from build123d import *

# Parameters (mm, degrees)
MODEL_R                 = 1.5
SALIENTE_EXTRUIR1_DEPTH = 3


with BuildPart() as part:
    # Model → Saliente-Extruir1 (new body)
    with BuildSketch(Plane.XY):
        Polygon((-105.943383637, 105.556539338), (-105.943383637, 51.556539338), (-51.943383637, 51.556539338), align=None)
        with Locations((-101.443383637, 92.056539338)):
            Circle(MODEL_R, mode=Mode.SUBTRACT)
        with Locations((-101.443383637, 83.056539338)):
            Circle(MODEL_R, mode=Mode.SUBTRACT)
        with Locations((-92.443383637, 83.056539338)):
            Circle(MODEL_R, mode=Mode.SUBTRACT)
        with Locations((-101.443383637, 74.056539338)):
            Circle(MODEL_R, mode=Mode.SUBTRACT)
        with Locations((-92.443383637, 74.056539338)):
            Circle(MODEL_R, mode=Mode.SUBTRACT)
        with Locations((-83.443383637, 74.056539338)):
            Circle(MODEL_R, mode=Mode.SUBTRACT)
        with Locations((-101.443383637, 65.056539338)):
            Circle(MODEL_R, mode=Mode.SUBTRACT)
        with Locations((-92.443383637, 65.056539338)):
            Circle(MODEL_R, mode=Mode.SUBTRACT)
        with Locations((-83.443383637, 65.056539338)):
            Circle(MODEL_R, mode=Mode.SUBTRACT)
        with Locations((-74.443383637, 65.056539338)):
            Circle(MODEL_R, mode=Mode.SUBTRACT)
        with Locations((-101.443383637, 56.056539338)):
            Circle(MODEL_R, mode=Mode.SUBTRACT)
        with Locations((-92.443383637, 56.056539338)):
            Circle(MODEL_R, mode=Mode.SUBTRACT)
        with Locations((-83.443383637, 56.056539338)):
            Circle(MODEL_R, mode=Mode.SUBTRACT)
        with Locations((-74.443383637, 56.056539338)):
            Circle(MODEL_R, mode=Mode.SUBTRACT)
        with Locations((-65.443383637, 56.056539338)):
            Circle(MODEL_R, mode=Mode.SUBTRACT)
    extrude(amount=SALIENTE_EXTRUIR1_DEPTH)


solid = part.part
Can you work these out from the model? Positions are in its coordinate system, mm. Round coordinates to 2 decimals unless told otherwise and drop trailing zeros. Order: outer loops, then holes, each group sorted by start corner. A loop starts at its lowest first (then second) coordinate and runs counter-clockwise, first axis right, second up. Notation, with made-up numbers: (82, -1.5) -> (93, -1.5) arc R14 ccw to (93, 20.5) -> close; hole circle Ø10 at (8.5, -36.5). An arc over 180 degrees is marked (long way). Write each question's results on one line, items separated by ' | '. Start each with the question number.
Item 1: If we section it at C-C, the plane z = 1.65: State how many separate pieces and enclosed holes the cut face has, then the cut area to 3 significant figures.
Item 2: Thinking about a two-plate mould opening in X: for faces 1 (the flat face through (-91, 67, 0)), 2 (the flat face through (-78.565, 78.179, 1.479)), 3 (the cylindrical face through (-100.8, 90.7, 1.5)), which applies, +X half, -X half, draft (parallel to the pull), parting line (faces both ways), or undercut?
Item 3: If we section it at A-A, the plane x = -65.5: Write out the boundary of the cut face in (y, z), then the cut area to 3 significant figures.
Item 4: If we section it at D-D, the plane x = -102: Write out the boundary of the cut face in (y, z).
Item 5: If we section it at B-B, the plane x = -74.5: Write out the boundary of the cut face in (y, z).
Item 6: Please list where these lines run through material, in increasing order: L1, parallel to X at y = 82, z = 0.3; L2, parallel to Y at x = -73.5, z = 1.4; L3, parallel to X at y = 74, z = 1.7.
Results:
1) separate pieces: 1 | enclosed holes: 15 | area: 1,350 mm2
2) face 1: draft | face 2: +X half | face 3: undercut
3) outline: (51.56, 0) -> (54.56, 0) -> (54.56, 3) -> (51.56, 3) -> close; (57.56, 0) -> (65.11, 0) -> (65.11, 3) -> (57.56, 3) -> close | area: 31.7 mm2
4) outline: (51.56, 0) -> (54.66, 0) -> (54.66, 3) -> (51.56, 3) -> close; (57.45, 0) -> (63.66, 0) -> (63.66, 3) -> (57.45, 3) -> close; (66.45, 0) -> (72.66, 0) -> (72.66, 3) -> (66.45, 3) -> close; (75.45, 0) -> (81.66, 0) -> (81.66, 3) -> (75.45, 3) -> close; (84.45, 0) -> (90.66, 0) -> (90.66, 3) -> (84.45, 3) -> close; (93.45, 0) -> (101.61, 0) -> (101.61, 3) -> (93.45, 3) -> close
5) outline: (51.56, 0) -> (54.56, 0) -> (54.56, 3) -> (51.56, 3) -> close; (57.56, 0) -> (63.56, 0) -> (63.56, 3) -> (57.56, 3) -> close; (66.56, 0) -> (74.11, 0) -> (74.11, 3) -> (66.56, 3) -> close
6) L1: x = -105.94 to -102.51, -100.38 to -93.51, -91.38 to -82.39 | L2: y = 51.56 to 54.89, 57.22 to 63.89, 66.22 to 73.11 | L3: x = -105.94 to -102.94, -99.94 to -93.94, -90.94 to -84.94, -81.94 to -74.39
